Verification items for this drawing (mm, ordinates from the low corner). A direction names the side the tool comes from. Give positions to 0.01 mm unless a question says otherwise; leave off trailing zeros. Write each loop counter-clockwise with the first axis right and the second up, starting at its lowest first coordinate (ties: lowest second). Pieces come first, ordered by that corner, then holes. Notation, with made-up numbers: M 2.5,-32 L 37.5,-32 A21 cw 37.5,-7 Z; hole C -26.5,-6.75 d6. An arc over 180 degrees is marked long. Write each question's results on one line, items separated by ' | '.
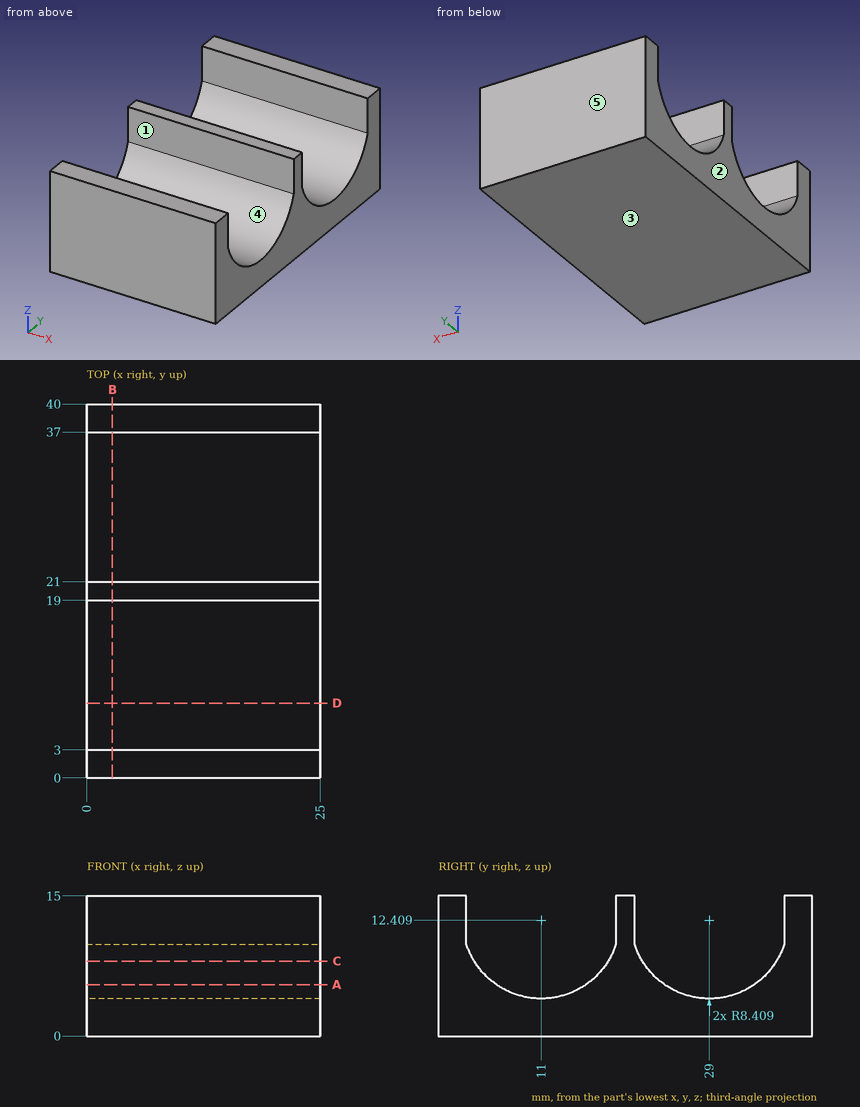
Q1. Section check D-D (y = 8). Enter the section's corners in (x, z), then the cut area to 3 significant figures.
Answer key:
outline: M 0,0 L 25,0 L 25,4.55 L 0,4.55 Z | area: 114 mm2
Q2. Release check for a two-part mould opening along Y. For the marked faces 3, 4 and 5 record: released by +Y, released by -Y, zero draft, split by the parting line, or undercut.
Answer key:
face 3: zero draft | face 4: undercut | face 5: released by +Y
Q3. Section check C-C (z = 8). Enter the section's corners in (x, y), then the cut area to 3 significant figures.
Answer key:
outline: M 0,0 L 25,0 L 25,3.84 L 0,3.84 Z; M 0,18.16 L 25,18.16 L 25,21.84 L 0,21.84 Z; M 0,36.16 L 25,36.16 L 25,40 L 0,40 Z | area: 284 mm2
Q4. Section check B-B (x = 2.75). Enter the section's corners in (y, z).
Answer key:
outline: M 0,0 L 40,0 L 40,15 L 37,15 L 37,9.82 A8.41 cw 21,9.82 L 21,15 L 19,15 L 19,9.82 A8.41 cw 3,9.82 L 3,15 L 0,15 Z
Q5. Section check A-A (z = 5.5). Enter the section's corners in (x, y), then the cut area to 3 significant figures.
Answer key:
outline: M 0,0 L 25,0 L 25,6.21 L 0,6.21 Z; M 0,15.79 L 25,15.79 L 25,24.21 L 0,24.21 Z; M 0,33.79 L 25,33.79 L 25,40 L 0,40 Z | area: 521 mm2
Q6. Depth check by flat-ended pin: P1, Ø3, axis at x = 9, y = 29, coming from the -Z side; P2, Ø8, axis at x = 6.5, y = 9, coming from the +Z side. Enter the tip coordinate at first touch or a pass-through.
Answer key:
P1: stops at z = 0 | P2: stops at z = 6.52
Q7. Material ranges on probe 1 along Y at (x, z) = (20.75, 13.75); probe 2 along Y at (x, z) = (5.75, 8.25); probe 3 along Z at (x, y) = (10, 12.5) (3 decimals), recorded low to high. Write a range as [from, to].
Answer key:
probe 1: y = [0, 3], [19, 21], [37, 40] | probe 2: y = [0, 3.69], [18.31, 21.69], [36.31, 40] | probe 3: z = [0, 4.135]
Q8. Access from +Z, -Z, +X, -X, +Y, -Y to the whole of each face (thin tool, end or side, straight path). Record for the marked faces 1 and 2.
Answer key:
face 1: +Z, +X, -X | face 2: +Z, -Z, -X, +Y, -Y
